Work out the finished part from the listing and answer in its coordinate system (mm). A direction names the side the tool comes from. Coordinates: 2 decimals unless noted, no trailing zeros. Order: outer loops, then holes, each group sorted by start corner. A loop starts at its lowest first (then second) coordinate and runs counter-clockwise, first axis right, second up. Notation, with made-up numbers: (52.5, 50) -> (74.5, 50) arc R23 ccw to (74.5, 84) -> close; hole circle Ø8 at (67, -6). An arc over 180 degrees is marked (long way). Answer as CSV lines item,"result". Start each with the question number.
Item 1: Which of the six approach directions +Z, -Z, +X, -X, +Y, -Y give full straight-line access (tool end or side, diameter ignored) to faces 1 (the face through (-30, 11, 1)), 2 (the face through (-22.5, 12, 1)), 3 (the face through (-1.745, 24.571, 2.014))?
Item 2: For a pull along Y with two mould halves and no side action, classify faces 4 (the face through (-0.05, 17.93, 1.48)), 5 (the face through (20.05, 17.93, 1.48)), 6 (the face through (-20.19, 53.09, 1.48)), 7 (the face through (0, 0, 1)) as pulls with the +Y half, pulls with the -Y half, needs draft (parallel to the pull), parting line crosses it, or undercut.
Item 3: Each of these flat-tipped pins is pushed along its axis until it touches: pin 1 Ø12.5 at (x, y) = (0, 32.43) entering from +Z; pin 2 Ø1.5 at (y, z) = (11.5, 1) entering from +X; pin 3 Ø0.9 at (y, z) = (12, 1.5) entering from -X. Where does it stop, or does it pass through?
Item 4: Section B-B (y = 32.43) is taken. Write down the section's boundary in (x, z), then the cut area to 3 significant figures.
Item 5: Section D-D (x = -7) is taken. Write down the section's boundary in (y, z).
Item 6: Section C-C (z = 2.2) is taken. Count the separate pieces of the cut face and the enclosed holes in it, then the cut area to 3 significant figures.
Item 7: Section A-A (x = 20) is taken. Write down the section's boundary in (y, z).
Item 8: Straight lines are drawn through the part: L1, parallel to Y at x = 0, z = 2.25; L2, parallel to X at y = 19.5, z = 2.1; L3, parallel to Y at x = 3, z = 1.7. For each, find the intervals that lie inside material, in ascending order.
```python
from build123d import *

# Parameters (mm, degrees)
MODEL_R             = 5.5
MODEL_R_2           = 2.5
BOSS_EXTRUDE1_DEPTH = 3
SKETCH2_R           = 8.05
CUT_EXTRUDE1_DEPTH  = 2


with BuildPart() as part:
    # Model → Boss-Extrude1 (new body)
    with BuildSketch(Plane.XY):
        with BuildLine():
            Line((-28.5, 0), (28.5, 0))
            ThreePointArc((28.5, 0), (29.560660172, 0.439339828), (30, 1.5))
            Line((30, 1.5), (30, 20.959120907))
            ThreePointArc((30, 20.959120907), (30.114180701, 21.533146056), (30.439339828, 22.019781079))
            Line((30.439339828, 22.019781079), (37.314024843, 28.894466094))
            ThreePointArc((37.314024843, 28.894466094), (38.778490937, 32.43), (37.314024843, 35.965533906))
            Line((37.314024843, 35.965533906), (3.535533906, 69.744024843))
            ThreePointArc((3.535533906, 69.744024843), (0, 71.208490937), (-3.535533906, 69.744024843))
            Line((-3.535533906, 69.744024843), (-37.314024843, 35.965533906))
            ThreePointArc((-37.314024843, 35.965533906), (-38.778490937, 32.43), (-37.314024843, 28.894466094))
            Line((-37.314024843, 28.894466094), (-30.439339828, 22.019781079))
            ThreePointArc((-30.439339828, 22.019781079), (-30.114180701, 21.533146056), (-30, 20.959120907))
            Line((-30, 20.959120907), (-30, 1.5))
            ThreePointArc((-30, 1.5), (-29.560660172, 0.439339828), (-28.5, 0))
        make_face()
        with Locations((0, 32.43)):
            Circle(MODEL_R, mode=Mode.SUBTRACT)
        with Locations((0, 65.76302733)):
            Circle(MODEL_R_2, mode=Mode.SUBTRACT)
        with Locations((33.333, 32.43)):
            Circle(MODEL_R_2, mode=Mode.SUBTRACT)
        with Locations((-33.333, 32.43)):
            Circle(MODEL_R_2, mode=Mode.SUBTRACT)
        with BuildLine():
            Line((22.5, 8.63), (22.5, 15.43))
            ThreePointArc((22.5, 15.43), (20, 17.93), (17.5, 15.43))
            Line((17.5, 15.43), (17.5, 8.63))
            ThreePointArc((17.5, 8.63), (20, 6.13), (22.5, 8.63))
        make_face(mode=Mode.SUBTRACT)
        with BuildLine():
            Line((-22.5, 8.63), (-22.5, 15.43))
            ThreePointArc((-22.5, 15.43), (-20, 17.93), (-17.5, 15.43))
            Line((-17.5, 15.43), (-17.5, 8.63))
            ThreePointArc((-17.5, 8.63), (-20, 6.13), (-22.5, 8.63))
        make_face(mode=Mode.SUBTRACT)
        with BuildLine():
            Line((-2.5, 8.63), (-2.5, 15.43))
            ThreePointArc((-2.5, 15.43), (0, 17.93), (2.5, 15.43))
            Line((2.5, 15.43), (2.5, 8.63))
            ThreePointArc((2.5, 8.63), (0, 6.13), (-2.5, 8.63))
        make_face(mode=Mode.SUBTRACT)
    extrude(amount=BOSS_EXTRUDE1_DEPTH)

    # Sketch2 → Cut-Extrude1 (cut)
    with BuildSketch(Plane.XY.offset(3)):
        with Locations((0, 32.43)):
            Circle(SKETCH2_R)
    extrude(amount=-CUT_EXTRUDE1_DEPTH, mode=Mode.SUBTRACT)


solid = part.part
```
Checked values:
1,face 1,"+Z, -Z, -X, -Y"
1,face 2,"+Z, -Z"
1,face 3,"+Z"
2,face 4,"undercut"
2,face 5,"undercut"
2,face 6,"pulls with the +Y half"
2,face 7,"pulls with the -Y half"
3,pin 1,"stops at z = 1"
3,pin 2,"stops at x = 30"
3,pin 3,"stops at x = -30"
4,outline,"(-38.78, 0) -> (-35.83, 0) -> (-35.83, 3) -> (-38.78, 3) -> close; (-30.83, 0) -> (-5.5, 0) -> (-5.5, 1) -> (-8.05, 1) -> (-8.05, 3) -> (-30.83, 3) -> close; (5.5, 0) -> (30.83, 0) -> (30.83, 3) -> (8.05, 3) -> (8.05, 1) -> (5.5, 1) -> close; (35.83, 0) -> (38.78, 0) -> (38.78, 3) -> (35.83, 3) -> close"
4,area,"159 mm^2"
5,outline,"(0, 0) -> (66.28, 0) -> (66.28, 3) -> (36.41, 3) -> (36.41, 1) -> (28.45, 1) -> (28.45, 3) -> (0, 3) -> close"
6,separate pieces,"1"
6,enclosed holes,"7"
6,area,"3,290 mm^2"
7,outline,"(0, 0) -> (6.13, 0) -> (6.13, 3) -> (0, 3) -> close; (17.93, 0) -> (53.28, 0) -> (53.28, 3) -> (17.93, 3) -> close"
8,L1,"y = 0 to 6.13, 17.93 to 24.38, 40.48 to 63.26, 68.26 to 71.21"
8,L2,"x = -30 to 30"
8,L3,"y = 0 to 24.96, 39.9 to 70.21"
